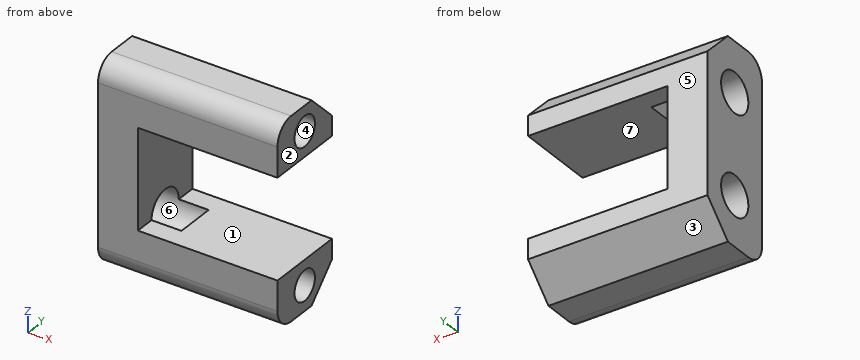
Autodesk Inventor part; units mm, degrees
ref_plane "YZ Plane" through (0, 0, 0) normal (1, 0, 0) x (0, 1, 0)
ref_plane "XZ Plane" through (0, 0, 0) normal (0, 1, 0) x (-1, 0, 0)
ref_plane "XY Plane" through (0, 0, 0) normal (0, 0, 1) x (1, 0, 0)
sketch "Sketch1" plane through (0, 0, 0) normal (0, 1, 0) x (-1, 0, 0)
  line L0 (0, 0) -> (18, 0)
  line L1 (18, 0) -> (18, -20)
  line L2 (18, -20) -> (0, -20)
  line L3 (0, -20) -> (0, 0)
  line L4 (0, 0) -> (0, -5)
  line L5 (0, -5) -> (14, -5)
  line L6 (14, -5) -> (14, -15)
  line L7 (14, -15) -> (0, -15)
  line L8 (0, -15) -> (0, -5)
  dimension "d0" = 18
  dimension "d1" = 20
  dimension "d2" = 5
  dimension "d3" = 14
  dimension "d4" = 10
extrude "Extrusion1" add sketch "Sketch1" along normal blind 8 contours L0 L1 L2 L3 L7 L6 L5
sketch "Sketch2" plane through (0, 0, 0) normal (1, 0, 0) x (0, 0, -1)
  line L0 (20, 8) -> (0, 8)
  line L1 (0, 8) -> (2.5, 8)
  line L2 (2.5, 8) -> (2.5, 4)
  line L3 (2.5, 4) -> (0, 4)
  line L4 (0, 4) -> (0, 8)
  line L5 (20, 0) -> (20, 8)
  line L6 (20, 8) -> (17.5, 8)
  line L7 (17.5, 8) -> (17.5, 4)
  line L8 (17.5, 4) -> (20, 4)
  line L9 (20, 4) -> (20, 8)
  circle A0 centre (2.5, 4) radius 1.5
  circle A1 centre (17.5, 4) radius 1.5
  point P0 (0, 0)
  dimension "d7" = 2.5
  dimension "d8" = 4
  dimension "d9" = 2.5
  dimension "d10" = 4
  dimension "d11" = 3
  dimension "d12" = 3
extrude "Extrusion2" cut sketch "Sketch2" against normal blind 7 contours A1 L8 L7 | L7 L8 A1 | A0 L3 L2 | L2 L3 A0
sketch "Sketch3" plane through (-18, 0, -20) normal (-1, 0, 0) x (0, 0, 1)
  line L0 (0, 0) -> (0, 8)
  line L1 (0, 0) -> (5, 0)
  line L2 (5, 0) -> (5, 4)
  line L3 (5, 4) -> (0, 4)
  line L4 (0, 4) -> (0, 0)
  line L5 (5, 4) -> (15, 4)
  circle A0 centre (5, 4) radius 2
  circle A1 centre (15, 4) radius 2
  point P0 (20, 0)
  dimension "d15" = 5
  dimension "d16" = 4
  dimension "d17" = 10
  dimension "d18" = 4
  dimension "d19" = 4
extrude "Extrusion3" cut sketch "Sketch3" against normal blind 7 contours A1 | A0 L5 L3 | L3 L2 A0 | L2 L5 A0
fillet "Fillet1" radius 2 2 edges at (-9, 0, 0) (-9, 0, -20)
chamfer "Chamfer1" distance 3 angle 45 2 edges at (-9, 8, -20) (-9, 8, 0)
properties part number "servo_support_4"
Part model, mm, in its own coordinate system. Face numbers are marked on the shaded views. A direction names the side the tool comes from. Round coordinates to 2 decimals unless told otherwise and drop trailing zeros. Loops run counter-clockwise (first coordinate to the right, second up) from the corner with the lowest first, then second, coordinate; pieces in that order, holes last.
1. Slice it at A-A (x = -6.75). Give the cut face in (y, z), and give its area (3 significant figures).
Solutions:
outline: (0, -18) arc R2 ccw to (2, -20) - (5, -20) - (8, -17) - (8, -15) - (0, -15) - close; (0, -5) - (8, -5) - (8, -3) - (5, 0) - (2, 0) arc R2 ccw to (0, -2) - close; hole circle Ø3 at (4, -17.5); hole circle Ø3 at (4, -2.5)
area: 55.1 mm2
2. Two-plate mould, pull along Z, no slides. Class the marked faces 1, 2 and 3: pulls with the +Z half, pulls with the -Z half, needs draft (parallel to the pull), parting line crosses it, or undercut.
Solutions:
face 1: undercut
face 2: needs draft
face 3: pulls with the -Z half
3. Slice it at D-D (y = 7). Give the cut face in (x, z).
Solutions:
outline: (-18, -18) - (0, -18) - (0, -15) - (-14, -15) - (-14, -5) - (0, -5) - (0, -2) - (-18, -2) - close
4. 3-axis set-ups, long thin cutter, end or side, ignore diameter. For the marked faces 4, 5, 6 and 7: which of +Z, -Z, +X, -X, +Y, -Y reach the whole face in a straight line?
Solutions:
face 4: +X
face 5: +Z, -Z, +X, -X, +Y
face 6: -X
face 7: +X, +Y, -Y
5. Drill centre lines: line 1 along Z through (x, y) = (-4.5, 4); line 2 along Z through (x, y) = (-14.5, 4.5); line 3 along Z through (x, y) = (-9.5, 3). Where is each one in solid material? Low to high.
Solutions:
line 1: z = -20 to -19, -16 to -15, -5 to -4, -1 to 0
line 2: z = -20 to -16.94, -13.06 to -6.94, -3.06 to 0
line 3: z = -20 to -15, -5 to 0
6. Slice it at C-C (y = 4). Give the cut face in (x, z).
Solutions:
outline: (-18, -20) - (0, -20) - (0, -19) - (-7, -19) - (-7, -16) - (0, -16) - (0, -15) - (-11, -15) - (-11, -17) - (-18, -17) - close; (-18, -13) - (-14, -13) - (-14, -7) - (-18, -7) - close; (-18, -3) - (-11, -3) - (-11, -5) - (0, -5) - (0, -4) - (-7, -4) - (-7, -1) - (0, -1) - (0, 0) - (-18, 0) - close
7. Flat gauge pins, fed straight in: pin 1 (2 mm diameter, centred on x = -7.5, z = -12.5, fed in from +Y); pin 2 (1.6 mm diameter, centred on y = 4, z = -16, fed in from -X); pin 3 (0.9 mm diameter, centred on y = 3.5, z = -2, fed in from +X); pin 4 (4 mm diameter, centred on y = 3, z = -11.5, fed in from +X). Where does each tip first touch, or does it go through?
Solutions:
pin 1: passes through
pin 2: stops at x = -11
pin 3: stops at x = -7
pin 4: stops at x = -14
8. Slice it at B-B (x = -12.25). Give the cut face in (y, z), and give its area (3 significant figures).
Solutions:
outline: (0, -18) arc R2 ccw to (2, -20) - (5, -20) - (8, -17) - (8, -15) - (6, -15) arc R2 cw to (2, -15) - (0, -15) - close; (0, -5) - (2, -5) arc R2 cw to (6, -5) - (8, -5) - (8, -3) - (5, 0) - (2, 0) arc R2 ccw to (0, -2) - close
area: 56.7 mm2
